Read the model definition and answer for the solid it produces. Units are mm, in the model's axes. A direction names the side the tool comes from. Round coordinates to 2 decimals unless told otherwise and drop trailing zeros. Order: outer loops, then holes, each group sorted by start corner. A loop starts at its lowest first (then second) coordinate and runs counter-clockwise, first axis right, second up. Notation, with made-up numbers: (-11, 79) -> (40, 79) arc R15 cw to (40, 93) -> close; hole circle Ø10 at (30.25, -35). An arc over 180 degrees is marked (long way). Use a Markdown table: item, result. Add a question column.
1. Section C-C, the plane z = 75 is taken. Give the vertices of the cut face in (x, y), then the cut area to 3 significant figures.
2. The mould has two halves that part along X. Classify faces 6 (the face through (-10, 25, 0)), 7 (the face through (880, 25, 74)), 8 (the face through (-775, 25, -600)): +X half, -X half, draft (parallel to the pull), parting line (faces both ways), or undercut.
3. Section B-B, the plane y = 41.5 is taken. Give the vertices of the cut face in (x, z).
4. Consider L1, parallel to X at y = 43, z = 75; L2, parallel to X at y = 32.5, z = -47; L3, parallel to X at y = 16, z = 93. Determine where each line is inside the solid, lowest interval first. Write a range as [from, to].
5. Given pin 1 (5 mm diameter, centred on y = 8, z = -401, fed in from +X); pin 2 (10 mm diameter, centred on x = -45, y = 42, fed in from -Z); pin 3 (6 mm diameter, centred on y = 37, z = -74.5, fed in from -X), each flat-ended and moving along its own axis, determine where each tip first touches the part or whether it passes through.
6. Section D-D, the plane x = -112.5 is taken. Give the vertices of the cut face in (y, z), then the cut area to 3 significant figures.
7. Section A-A, the plane z = -89 is taken. Give the vertices of the cut face in (x, y), then the cut area to 3 significant figures.
8. For faces 1 (the face through (12, 0, 30)), 2 (the face through (835, 25, 0)), 3 (the face through (-800, 25, -296)), 4 (the face through (-781.324, 12.325, 103.724)), 5 (the face through (750, 25, -296)), determine the directions among +Z, -Z, +X, -X, +Y, -Y from which every point of the face is accessible in a straight line to the end or side of a thin tool.
Autodesk Inventor part; units mm, degrees
ref_plane "YZ Plane" through (0, 0, 0) normal (1, 0, 0) x (0, 1, 0)
ref_plane "XZ Plane" through (0, 0, 0) normal (0, 1, 0) x (-1, 0, 0)
ref_plane "XY Plane" through (0, 0, 0) normal (0, 0, 1) x (1, 0, 0)
sketch "Skizze1" plane through (0, 0, 0) normal (0, 1, 0) x (-1, 0, 0)
  line L0 (800, 0) -> (800, -600)
  line L1 (800, -600) -> (750, -600)
  line L2 (750, -600) -> (750, 0)
  line L3 (750, 0) -> (-750, 0)
  line L4 (-750, 0) -> (-750, -600)
  line L5 (-750, -600) -> (-800, -600)
  line L6 (-800, -600) -> (-800, 0)
  line L7 (-800, 0) -> (-880, 0)
  line L8 (-880, 0) -> (-880, 150)
  line L9 (-880, 150) -> (880, 150)
  line L10 (880, 150) -> (880, 0)
  line L11 (880, 0) -> (800, 0)
  line L12 (0, -750) -> (0, 300)
  point P0 (0, 0)
  dimension "d0" = 50
  dimension "d1" = 600
  dimension "d2" = 150
  dimension "d3" = 1500
  dimension "d4" = 80
extrude "Extrusion1" add sketch "Skizze1" along normal blind 50
sketch "Skizze2" plane through (0, 0, 0) normal (0, -1, 0) x (1, 0, 0)
  circle A0 centre (-750, 75) radius 42.5
  circle A1 centre (750, 75) radius 42.5
  line L0 (0, -750) -> (0, 300)
  line L1 (750, 0) -> (-750, 0)
  point P0 (0, 0)
  dimension "d7" = 85
  dimension "d8" = 85
  dimension "d9" = 1500
  dimension "d10" = 75
extrude "Extrusion2" cut sketch "Skizze2" against normal blind 25
sketch "Skizze3" plane through (0, 50, 0) normal (0, 1, 0) x (1, 0, 0)
  circle A0 centre (750, -75) radius 42.5
  circle A1 centre (-750, -75) radius 42.5
  circle A2 centre (750, -75) radius 17.5
  circle A3 centre (-750, -75) radius 17.5
  point P0 (0, 0)
  dimension "d13" = 35
  dimension "d14" = 35
extrude "Extrusion3" cut sketch "Skizze3" against normal through all contours A2 | A3
chamfer "Fase1" distance 10 angle 45 4 edges at (-880, 25, 150) (880, 25, 150) (880, 25, 0) (-880, 25, 0)
equation "\"d8\" = d7"
properties part number "Gestell_Seite"
Verdict:
| question | item | result |
|---|---|---|
| 1 | outline | (-880, 0) -> (-792.5, 0) -> (-792.5, 25) -> (-767.5, 25) -> (-767.5, 50) -> (-880, 50) -> close; (-732.5, 25) -> (-707.5, 25) -> (-707.5, 0) -> (707.5, 0) -> (707.5, 25) -> (732.5, 25) -> (732.5, 50) -> (-732.5, 50) -> close; (767.5, 25) -> (792.5, 25) -> (792.5, 0) -> (880, 0) -> (880, 50) -> (767.5, 50) -> close |
| 1 | area | 82,000 mm2 |
| 2 | face 6 | undercut |
| 2 | face 7 | +X half |
| 2 | face 8 | draft |
| 3 | outline | (-880, 10) -> (-870, 0) -> (-800, 0) -> (-800, -600) -> (-750, -600) -> (-750, 0) -> (750, 0) -> (750, -600) -> (800, -600) -> (800, 0) -> (870, 0) -> (880, 10) -> (880, 140) -> (870, 150) -> (-870, 150) -> (-880, 140) -> close; hole circle Ø35 at (-750, 75); hole circle Ø35 at (750, 75) |
| 4 | L1 | x = [-880, -767.5], [-732.5, 732.5], [767.5, 880] |
| 4 | L2 | x = [-800, -750], [750, 800] |
| 4 | L3 | x = [-880, -788.5], [-711.5, 711.5], [788.5, 880] |
| 5 | pin 1 | stops at x = 800 |
| 5 | pin 2 | stops at z = 0 |
| 5 | pin 3 | stops at x = -800 |
| 6 | outline | (0, 0) -> (50, 0) -> (50, 150) -> (0, 150) -> close |
| 6 | area | 7,500 mm2 |
| 7 | outline | (-800, 0) -> (-750, 0) -> (-750, 50) -> (-800, 50) -> close; (750, 0) -> (800, 0) -> (800, 50) -> (750, 50) -> close |
| 7 | area | 5,000 mm2 |
| 8 | face 1 | +Z, -Z, +X, -X, -Y |
| 8 | face 2 | -Z, +X, +Y, -Y |
| 8 | face 3 | -Z, -X, +Y, -Y |
| 8 | face 4 | -Y |
| 8 | face 5 | -Z, +Y, -Y |
